```python
from build123d import *

# Parameters (mm, degrees)
SKETCH_1_W          = 100
SKETCH_1_H          = 68
EXTRUDE_1_DEPTH     = 3
SKETCH_2_W          = 100
SKETCH_2_H          = 3
EXTRUDE_2_DEPTH     = 27
SKETCH_3_W          = 7
SKETCH_3_H          = 24
CUT_EXTRUDE_2_DEPTH = 27
SKETCH_4_W          = 62
SKETCH_4_H          = 5
EXTRUDE_3_DEPTH     = 52
SKETCH_5_R          = 1.5
CUT_EXTRUDE_4_DEPTH = 5
SKETCH_7_W          = 35
SKETCH_7_H          = 48
CUT_EXTRUDE_5_DEPTH = 3
SKETCH_8_W          = 55
SKETCH_8_H          = 3
EXTRUDE_4_DEPTH     = 45
SKETCH_10_R         = 2
SKETCH_10_W         = 32
SKETCH_10_H         = 36
CUT_EXTRUDE_6_DEPTH = 45
SKETCH_12_R         = 3
CUT_EXTRUDE_7_DEPTH = 2
SKETCH_13_W         = 40
SKETCH_13_H         = 27
CUT_EXTRUDE_8_DEPTH = 10
FILLET_1_R          = 20


with BuildPart() as part:
    # 스케치1 → 보스-돌출1 (new body)
    with BuildSketch(Plane(origin=(0, 0, 0), x_dir=(1, 0, 0), z_dir=(0, 1, 0))):
        Rectangle(SKETCH_1_W, SKETCH_1_H)
    extrude(amount=EXTRUDE_1_DEPTH)

    # 스케치2 → 보스-돌출2 (add)
    with BuildSketch(Plane(origin=(0, 3, 0), x_dir=(1, 0, 0), z_dir=(0, 1, 0))):
        with Locations((0, 32.5)):
            Rectangle(SKETCH_2_W, SKETCH_2_H)
    extrude(amount=EXTRUDE_2_DEPTH)

    # 스케치3 → 컷-돌출2 (cut)
    with BuildSketch(Plane.XY.offset(-31)):
        with Locations((-35, 15)):
            Rectangle(SKETCH_3_W, SKETCH_3_H)
        with Locations((35, 15)):
            Rectangle(SKETCH_3_W, SKETCH_3_H)
    extrude(amount=-CUT_EXTRUDE_2_DEPTH, mode=Mode.SUBTRACT)

    # 스케치4 → 보스-돌출3 (add)
    with BuildSketch(Plane(origin=(0, 3, 0), x_dir=(1, 0, 0), z_dir=(0, 1, 0))):
        with Locations((0, -31.5)):
            Rectangle(SKETCH_4_W, SKETCH_4_H)
    extrude(amount=EXTRUDE_3_DEPTH)

    # 스케치5 → 컷-돌출4 (cut)
    with BuildSketch(Plane.XY.offset(34)):
        with Locations((-23, 30)):
            Circle(SKETCH_5_R)
        with Locations((23, 30)):
            Circle(SKETCH_5_R)
        with BuildLine():
            Line((-15, 30), (-15, 3))
            Line((-15, 3), (15, 3))
            Line((15, 3), (15, 30))
            ThreePointArc((15, 30), (0, 45), (-15, 30))
        make_face()
    extrude(amount=-CUT_EXTRUDE_4_DEPTH, mode=Mode.SUBTRACT)

    # 스케치7 → 컷-돌출5 (cut)
    with BuildSketch(Plane.XZ):
        with Locations((22.5, 0)):
            Rectangle(SKETCH_7_W, SKETCH_7_H)
        with Locations((-22.5, 0)):
            Rectangle(SKETCH_7_W, SKETCH_7_H)
    extrude(amount=-CUT_EXTRUDE_5_DEPTH, mode=Mode.SUBTRACT)

    # 스케치8 → 보스-돌출4 (add)
    with BuildSketch(Plane(origin=(50, 0, 0), x_dir=(0, 0, -1), z_dir=(1, 0, 0))):
        with Locations((6.5, 1.5)):
            Rectangle(SKETCH_8_W, SKETCH_8_H)
    extrude(amount=EXTRUDE_4_DEPTH)

    # 스케치10 → 컷-돌출6 (cut)
    with BuildSketch(Plane(origin=(0, 3, 0), x_dir=(1, 0, 0), z_dir=(0, 1, 0))):
        with Locations((55.5, -15.5)):
            Circle(SKETCH_10_R)
        with Locations((55.5, 28.5)):
            Circle(SKETCH_10_R)
        with Locations((89.5, 28.5)):
            Circle(SKETCH_10_R)
        with Locations((89.5, -15.5)):
            Circle(SKETCH_10_R)
        with Locations((72.5, 6.5)):
            Rectangle(SKETCH_10_W, SKETCH_10_H)
    extrude(amount=-CUT_EXTRUDE_6_DEPTH, mode=Mode.SUBTRACT)

    # 스케치12 → 컷-돌출7 (cut)
    with BuildSketch(Plane.XZ):
        with Locations((89.5, -28.5)):
            Circle(SKETCH_12_R)
        with Locations((89.5, 15.5)):
            Circle(SKETCH_12_R)
        with Locations((55.5, 15.5)):
            Circle(SKETCH_12_R)
        with Locations((55.5, -28.5)):
            Circle(SKETCH_12_R)
    extrude(amount=-CUT_EXTRUDE_7_DEPTH, mode=Mode.SUBTRACT)

    # 스케치13 → 컷-돌출8 (cut)
    with BuildSketch(Plane(origin=(0, 0, -34), x_dir=(-1, 0, 0), z_dir=(0, 0, -1))):
        with Locations((0, 16.5)):
            Rectangle(SKETCH_13_W, SKETCH_13_H)
    extrude(amount=-CUT_EXTRUDE_8_DEPTH, mode=Mode.SUBTRACT)

    # 필렛1
    fillet_1_edges = [part.edges().sort_by_distance(p)[0] for p in [
        (31, 55, 31.5),
        (-31, 55, 31.5),
    ]]
    fillet(fillet_1_edges, radius=FILLET_1_R)


solid = part.part
```
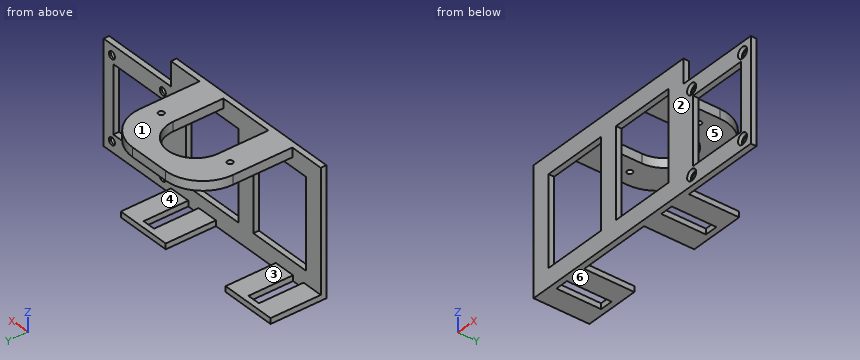
Part model, mm, in its own coordinate system. Face numbers are marked on the shaded views. A direction names the side the tool comes from. Give positions to 0.01 mm unless a question says otherwise; leave off trailing zeros. Loops run counter-clockwise (first coordinate to the right, second up) from the corner with the lowest first, then second, coordinate; pieces in that order, holes last. Notation, with made-up numbers: M -4,77.5 L 23,77.5 A15 cw 23,96.5 Z; hole C -35,87 d2. An arc over 180 degrees is marked long. Return JSON: item names as keys, results as strings.
1) Drill centre lines: line 1 (X direction, y = 2.3, z = 15.5); line 2 (Z direction, x = 89.5, y = 0.75); line 3 (Z direction, x = 55.5, y = 2.35). Where is each one in solid material? Low to high.
Calculated:
{"line 1": "x = -50 to -40, -5 to 5, 40 to 53.5, 57.5 to 87.5, 91.5 to 95", "line 2": "z = -34 to -31.5, -25.5 to 12.5, 18.5 to 21", "line 3": "z = -34 to -30.5, -26.5 to 13.5, 17.5 to 21"}
2) Pull direction Z, two halves, no side cores. Call the marked faces 1, 2, 3 and 4: released by +Z, released by -Z, zero draft, split by the parting line, or undercut.
Calculated:
{"face 1": "released by +Z", "face 2": "zero draft", "face 3": "undercut", "face 4": "undercut"}
3) Saw through at A-A, the plane z = -28.5. List the corners of the cut face in (x, y).
Calculated:
{"outline": "M -50,0 L 52.5,0 L 52.5,2 L 53.5,2 L 53.5,3 L -50,3 Z; M 57.5,2 L 58.5,2 L 58.5,0 L 86.5,0 L 86.5,2 L 87.5,2 L 87.5,3 L 57.5,3 Z; M 91.5,2 L 92.5,2 L 92.5,0 L 95,0 L 95,3 L 91.5,3 Z"}
4) 3-axis set-ups, long thin cutter, end or side, ignore diameter. For the marked faces 5 and 6: which of +Z, -Z, +X, -X, +Y, -Y reach the whole face in a straight line?
Calculated:
{"face 5": "+X, -X, +Y", "face 6": "-Z, +X, -X, +Y, -Y"}
5) Flat gauge pins, fed straight in: pin 1 Ø2.5 at (y, z) = (13.5, -33) entering from +X; pin 2 Ø4 at (y, z) = (17.5, 32) entering from -X; pin 3 Ø2.5 at (x, y) = (69, 1.5) entering from +Z. Where does each tip first touch, or does it go through?
Calculated:
{"pin 1": "stops at x = 50", "pin 2": "stops at x = -31", "pin 3": "stops at z = 21"}
6) Saw through at C-C, the plane x = 73.5. List the corners of the cut face in (y, z), then the cut area to 3 significant figures.
Calculated:
{"outline": "M 0,-34 L 3,-34 L 3,-24.5 L 0,-24.5 Z; M 0,11.5 L 3,11.5 L 3,21 L 0,21 Z", "area": "57.0 mm2"}
7) Saw through at D-D, the plane x = -23. List the corners of the cut face in (y, z).
Calculated:
{"outline": "M 0,-34 L 30,-34 L 30,-31 L 3,-31 L 3,-24 L 0,-24 Z; M 0,24 L 3,24 L 3,29 L 28.5,29 L 28.5,34 L 0,34 Z; M 31.5,29 L 51,29 L 51,34 L 31.5,34 Z"}
8) Saw through at B-B, the plane y = 25. List the corners of the cut face in (x, z).
Calculated:
{"outline": "M -50,-34 L -38.5,-34 L -38.5,-31 L -50,-31 Z; M -31.5,-34 L -20,-34 L -20,-31 L -31.5,-31 Z; M -31,29 L -15,29 L -15,34 L -31,34 Z; M 15,29 L 31,29 L 31,34 L 15,34 Z; M 20,-34 L 31.5,-34 L 31.5,-31 L 20,-31 Z; M 38.5,-34 L 50,-34 L 50,-31 L 38.5,-31 Z"}
